The model under review builds one solid part; all positions refer to its coordinate system, in mm. A direction names the side the tool comes from. Coordinates: 2 decimals unless noted, no trailing zeros. Write each loop counter-clockwise with the first axis right and the second up, starting at its lowest first coordinate (ties: lowest second). Pieces come first, ordered by that corner, then holes. Notation, with made-up numbers: (-10.75, 55) -> (0.25, 55) arc R14 cw to (0.25, 63) -> close; hole circle Ø5 at (22, -20.75). An arc over 180 degrees is marked (long way). Put each result on its own line as item: value. Start each with the question number.
Autodesk Inventor part; units mm, degrees
ref_plane "YZ Plane" through (0, 0, 0) normal (1, 0, 0) x (0, 1, 0)
ref_plane "XZ Plane" through (0, 0, 0) normal (0, 1, 0) x (-1, 0, 0)
ref_plane "XY Plane" through (0, 0, 0) normal (0, 0, 1) x (1, 0, 0)
sketch "スケッチ1" plane through (0, 0, 0) normal (1, 0, 0) x (0, 1, 0)
  circle A0 centre (0, 0) radius 5
  circle A1 centre (0, -35) radius 5
  line L0 (0, 0) -> (0, -35)
  circle A2 centre (0, -17.5) radius 12.5
  circle A3 centre (0, -17.5) radius 22.5
  point P0 (0, 5)
  point P1 (0, -5)
  point P2 (0, -30)
  point P3 (0, -40)
  dimension "d0" = 10
  dimension "d1" = 10
  dimension "d2" = 35
extrude "押し出し1" add sketch "スケッチ1" along normal blind 3 contours A0 | A0 A3 A1 A2 | A1 picked at (8.8989, -32.0838)
sketch "スケッチ2" plane through (3, 0, 0) normal (1, 0, 0) x (0, 0, -1)
  arc A0 (30, 0) -> (40, 0) centre (35, 0) ccw
  circle A1 centre (35, 0) radius 5
  point P0 (0, 0)
  point P1 (40, 0)
  point P2 (30, 0)
  dimension "d5" = 10
extrude "押し出し2" add sketch "スケッチ2" along normal blind 3
sketch "スケッチ3" plane through (0, 0, 0) normal (-1, 0, 0) x (0, 0, 1)
  arc A0 (-40, 0) -> (-30, 0) centre (-35, 0) ccw
  arc A1 (-5, 0) -> (5, 0) centre (0, 0) ccw
hole "穴1" at (0, 0, -35) at (0, 0, 0) direction (1, 0, 0) diameter 3.2 end through all
sketch "スケッチ4" plane through (0, 0, 0) normal (-1, 0, 0) x (0, 0, 1)
  circle A0 centre (-35, 0) radius 1.6
  circle A1 centre (-35, 0) radius 3.5
  point P0 (0, 0)
  dimension "d15" = 7
extrude "押し出し3" cut sketch "スケッチ4" against normal blind 4
properties part number "endeff_3dp3" material "ABS プラスチック"
1. Tool access review of faces 1 (the cylindrical face through (1.972, 0.154, -38.497)), 2 (the cylindrical face through (1.52, 0.97, -1.27)): name each direction out of +Z, -Z, +X, -X, +Y, -Y from which nothing blocks a thin tool from reaching the whole face with its end or side.
2. Consider section B-B on y = 7.5. State the section outline as (x, z) points.
3. Wall thickness on line 1 (Z direction, x = 5.15, y = 0); line 2 (Y direction, x = 5.2, z = -35); line 3 (Y direction, x = 3.1, z = -35): over which ranges is each line inside the solid? List them lowest first. Write a range as from..to.
4. Insertion check: P1, Ø5, axis at y = 0, z = -35, coming from the +X side; P2, Ø3.5, axis at y = 1.5, z = -35, coming from the -X side; P3, Ø12, axis at y = 11, z = -24.5, coming from the +X side; P4, Ø1, axis at x = 2, z = -5.5, coming from the +Y side. Each pin has a flat end and moves straight along its axis. Give the tip position at first contact, or say it passes through.
5. Consider section A-A on x = 1.05. State the section outline as (y, z) points.
6. The part is to be moulded in two halves that separate along Y. For faces 3 (the flat face through (0, 12, -12)), 4 (the cylindrical face through (3.625, -4.957, -34.349)), 5 (the flat face through (4, -2, -34)), say which applies: released by +Y, released by -Y, zero draft, split by the parting line, or undercut.
7. Consider section C-C on z = -35. State the section outline as (x, y) points.
8. Consider section D-D on x = 4.55. State the section outline as (y, z) points, then the cut area to 3 significant figures.
Output values:
1. face 1: -X
1. face 2: +X, -X
2. outline: (0, -38.71) -> (3, -38.71) -> (3, -27.5) -> (0, -27.5) -> close; (0, -7.5) -> (3, -7.5) -> (3, 3.71) -> (0, 3.71) -> close
3. line 1: z = -40..-36.6, -33.4..-30
3. line 2: y = -5..-1.6, 1.6..5
3. line 3: y = -5..-3.5, 3.5..5
4. P1: stops at x = 6
4. P2: stops at x = 4
4. P3: stops at x = 3
4. P4: stops at y = 19.34
5. outline: (0, -40) arc R22.5 ccw to (0, 5) arc R5 ccw to (0, -5) arc R12.5 cw to (0, -30) arc R5 ccw to start; hole circle Ø7 at (0, -35); hole circle Ø3.2 at (0, 0)
6. face 3: zero draft
6. face 4: split by the parting line
6. face 5: undercut
7. outline: (0, -5) -> (6, -5) -> (6, -1.6) -> (4, -1.6) -> (4, -3.5) -> (0, -3.5) -> close; (0, 3.5) -> (4, 3.5) -> (4, 1.6) -> (6, 1.6) -> (6, 5) -> (3, 5) -> (3, 14.14) -> (0, 14.14) -> close
8. outline: circle Ø10 at (0, -35); hole circle Ø3.2 at (0, -35)
8. area: 70.5 mm^2
